```python
from build123d import *

# Parameters (mm, degrees)
F0_R     = 9.525
F1_DEPTH = 25.4
F2_R     = 4.515684
F3_DEPTH = 25.401
F2_W     = 9.515054
F2_H     = 9.525
F4_DEPTH = 11.0998
F5_R     = 4.515684
F6_DEPTH = 9.525


with BuildPart() as f1:
    # F0 (on Front) → F1 (new body)
    with BuildSketch(Plane.XZ):
        Circle(F0_R)
    extrude(amount=F1_DEPTH)

    # F2 (on Front) → F3 (cut, through all)
    with BuildSketch(Plane.XZ):
        Circle(F2_R)
    extrude(amount=F3_DEPTH, mode=Mode.SUBTRACT)

    # F2 (on Front) → F4 (cut)
    with BuildSketch(Plane.XZ):
        Rectangle(F2_W, F2_H)
        Circle(F2_R, mode=Mode.SUBTRACT)
    extrude(amount=F4_DEPTH, mode=Mode.SUBTRACT)

    # F5 (on face) → F6 (cut)
    with BuildSketch(Plane.XZ.offset(25.4)):
        Polygon((-0.856141, 7.25214), (-6.708608, 2.88463), (-5.852467, -4.36751), (0.856141, -7.25214), (6.708608, -2.88463), (5.852467, 4.36751), align=None)
        Circle(F5_R, mode=Mode.SUBTRACT)
    extrude(amount=-F6_DEPTH, mode=Mode.SUBTRACT)


solid = f1.part
```
The listing builds one solid part. Answer for the finished solid, in the listing's coordinates (mm). A direction names the side the tool comes from. Give positions to 0.01 mm unless a question says otherwise; leave off trailing zeros. Order: outer loops, then holes, each group sorted by start corner. A loop starts at its lowest first (then second) coordinate and runs counter-clockwise, first axis right, second up. Notation, with made-up numbers: (44, -20) -> (85, -20) arc R22 ccw to (85, -5) -> close; hole circle Ø3 at (21.5, 42.5). An arc over 180 degrees is marked (long way). Answer as a JSON object with one key per item and string values. Group by question number.
Item 1: The part is cut by section A-A on z = 0. Write down the section's boundary in (x, y) (3 decimals).
Item 2: Determine the mould class of faces 1 (the flat face through (0, 0, -6)), 2 (the flat face through (-3.74, -20.7, 5.1)), 3 (the cylindrical face through (-7.559, -12.522, -5.796)) for opening direction Z: pulls with the +Z half, pulls with the -Z half, needs draft (parallel to the pull), parting line crosses it, or undercut.
Item 3: A tool of negligible diameter and unlimited length cuts with its end or side. For faces 4 (the flat face through (4.758, -5, 0)), 5 (the flat face through (3.74, -20.7, -5.1)), 6 (the cylindrical face through (4.307, -13.454, 1.356)), from which of +Z, -Z, +X, -X, +Y, -Y can it reach the whole face along a straight path? Write none if from no direction.
Item 4: Consider L1, parallel to Z at x = 0, y = -13.9 (3 decimals); L2, parallel to X at y = -18, z = -7; L3, parallel to Y at x = -5.25, z = 0.5 (3 decimals). Determine where each line is inside the solid, lowest interval first. Write a range as from..to.
Item 5: The part is cut by section D-D on z = -5.25. Write down the section's boundary in (x, y) (3 decimals), and give its area (3 significant figures).
Item 6: The part is cut by section C-C on y = -22.5. Write down the section's boundary in (x, z) (3 decimals), and give its area (3 significant figures).
Item 7: Flat-ended cylindrical pins translate along their axes: pin 1 (5 mm diameter, centred on x = -0.5, z = 6.5, fed in from -Y); pin 2 (6.5 mm diameter, centred on x = 2, z = -1.5, fed in from -Y) (3 decimals); pin 3 (1 mm diameter, centred on y = -5, z = 4.5, fed in from -X); pin 4 (4 mm diameter, centred on y = -10, z = -5.5, fed in from +X). Find the tip coordinate at first contact, or state that the pin passes through.
Result set:
{
 "1": {"outline": "(-9.525, -25.4) -> (-6.368, -25.4) -> (-6.368, -15.875) -> (-4.516, -15.875) -> (-4.516, -11.1) -> (-4.758, -11.1) -> (-4.758, 0) -> (-9.525, 0) -> close; (4.516, -15.875) -> (6.368, -15.875) -> (6.368, -25.4) -> (9.525, -25.4) -> (9.525, 0) -> (4.758, 0) -> (4.758, -11.1) -> (4.516, -11.1) -> close"},
 "2": {"face 1": "needs draft", "face 2": "undercut", "face 3": "parting line crosses it"},
 "3": {"face 4": "+Y", "face 5": "-Y", "face 6": "+Y, -Y"},
 "4": {"L1": "-9.525..-4.516, 4.516..9.525", "L2": "-6.46..0.27, 1.19..6.46", "L3": "-15.875..0"},
 "5": {"outline": "(-7.948, -25.4) -> (-3.8, -25.4) -> (-3.8, -15.875) -> (3.539, -15.875) -> (3.539, -25.4) -> (7.948, -25.4) -> (7.948, 0) -> (-7.948, 0) -> close", "area": "334 mm²"},
 "6": {"outline": "circle Ø19.05 at (0, 0); hole (-6.709, 2.885) -> (-5.852, -4.368) -> (0.856, -7.252) -> (6.709, -2.885) -> (5.852, 4.368) -> (-0.856, 7.252) -> close", "area": "146 mm²"},
 "7": {"pin 1": "y = -25.4", "pin 2": "y = -15.875", "pin 3": "x = -8.64", "pin 4": "x = 8.86"}
}
